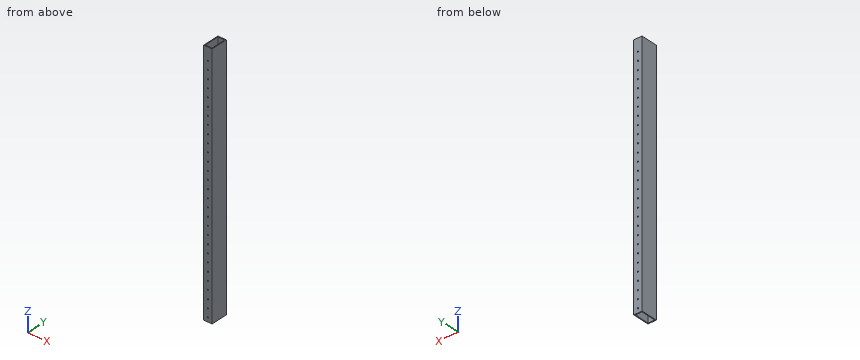
Autodesk Inventor part; units mm, degrees
ref_plane "YZ Plane" through (0, 0, 0) normal (1, 0, 0) x (0, 1, 0)
ref_plane "XZ Plane" through (0, 0, 0) normal (0, 1, 0) x (-1, 0, 0)
ref_plane "XY Plane" through (0, 0, 0) normal (0, 0, 1) x (1, 0, 0)
sketch "Sketch1" plane through (0, 0, 0) normal (0, 0, 1) x (1, 0, 0)
  line L0 (0, 0) -> (25.4, 0)
  line L1 (25.4, 0) -> (25.4, 50.8)
  line L2 (25.4, 50.8) -> (0, 50.8)
  line L3 (0, 50.8) -> (0, 0)
  line L4 (22.86, 48.26) -> (22.86, 2.54)
  line L5 (22.86, 2.54) -> (2.54, 2.54)
  line L6 (2.54, 2.54) -> (2.54, 48.26)
  line L7 (2.54, 48.26) -> (22.86, 48.26)
  dimension "d0" = 25.4
  dimension "d1" = 50.8
  dimension "d2" = 2.54
extrude "Extrusion1" add sketch "Sketch1" along normal blind 762
sketch "Sketch2" plane through (0, 50.8, 0) normal (0, 1, 0) x (1, 0, 0)
  circle A0 centre (12.7, -12.7) radius 1.9844
  line L0 (25.4, 0) -> (0, 0)
  line L1 (0, 0) -> (0, -762)
  circle A1 centre (12.7, -38.1) radius 1.9844
  circle A2 centre (12.7, -63.5) radius 1.9844
  circle A3 centre (12.7, -88.9) radius 1.9844
  circle A4 centre (12.7, -114.3) radius 1.9844
  circle A5 centre (12.7, -139.7) radius 1.9844
  circle A6 centre (12.7, -165.1) radius 1.9844
  circle A7 centre (12.7, -190.5) radius 1.9844
  circle A8 centre (12.7, -215.9) radius 1.9844
  circle A9 centre (12.7, -241.3) radius 1.9844
  circle A10 centre (12.7, -266.7) radius 1.9844
  circle A11 centre (12.7, -292.1) radius 1.9844
  circle A12 centre (12.7, -317.5) radius 1.9844
  circle A13 centre (12.7, -342.9) radius 1.9844
  circle A14 centre (12.7, -368.3) radius 1.9844
  circle A15 centre (12.7, -393.7) radius 1.9844
  circle A16 centre (12.7, -419.1) radius 1.9844
  circle A17 centre (12.7, -444.5) radius 1.9844
  circle A18 centre (12.7, -469.9) radius 1.9844
  circle A19 centre (12.7, -495.3) radius 1.9844
  circle A20 centre (12.7, -520.7) radius 1.9844
  circle A21 centre (12.7, -546.1) radius 1.9844
  circle A22 centre (12.7, -571.5) radius 1.9844
  circle A23 centre (12.7, -596.9) radius 1.9844
  circle A24 centre (12.7, -622.3) radius 1.9844
  circle A25 centre (12.7, -647.7) radius 1.9844
  circle A26 centre (12.7, -673.1) radius 1.9844
  circle A27 centre (12.7, -698.5) radius 1.9844
  circle A28 centre (12.7, -723.9) radius 1.9844
  circle A29 centre (12.7, -749.3) radius 1.9844
  circle A30 centre (12.7, -774.7) radius 1.9844
  circle A31 centre (12.7, -800.1) radius 1.9844
  circle A32 centre (12.7, -825.5) radius 1.9844
  dimension "d5" = 3.9688
  dimension "d6" = 12.7
  dimension "d7" = 12.7
  dimension "d10" = 25.4
extrude "Extrusion2" cut sketch "Sketch2" against normal blind 558.8 contours A0 | A1 | A2 | A3 | A4 | A5 | A6 | A7 | A8 | A9 | A10 | A11 | A12 | A13 | A14 | A15 | A16 | A17 | A18 | A19 | A20 | A21 | A22 | A23 | A24 | A25 | A26 | A27 | A28 | A30 | A31 | A32
properties part number "30in OChannel 1x2" material "Aluminum 6061-AHC"
Read the model definition and answer for the solid it produces. Units are mm, in the model's axes. Give positions to 0.01 mm unless a question says otherwise; leave off trailing zeros. Loops run counter-clockwise (first coordinate to the right, second up) from the corner with the lowest first, then second, coordinate; pieces in that order, holes last. Notation, with made-up numbers: M 77,34 L 121,34 A8 cw 121,40 Z; hole C 65.5,89.5 d10. An arc over 180 degrees is marked long. Write each question's results on one line, items separated by ' | '.
1. Given pin 1 (6.5 mm diameter, centred on x = 12.7, z = 38.1, fed in from -Y); pin 2 (3 mm diameter, centred on x = 12.7, z = 520.7, fed in from -Y), each flat-ended and moving along its own axis, determine where each tip first touches the part or whether it passes through.
Values:
pin 1: stops at y = 0 | pin 2: passes through
2. Section A-A on z = 632.5 is taken. Give the vertices of the cut face in (x, y), plus the area to 3 significant figures.
Values:
outline: M 0,0 L 25.4,0 L 25.4,50.8 L 0,50.8 Z; hole M 2.54,2.54 L 22.86,2.54 L 22.86,48.26 L 2.54,48.26 Z | area: 361 mm^2
3. Section B-B on y = 9.5 is taken. Give the vertices of the cut face in (x, z), plus the area to 3 significant figures.
Values:
outline: M 0,0 L 2.54,0 L 2.54,762 L 0,762 Z; M 22.86,0 L 25.4,0 L 25.4,762 L 22.86,762 Z | area: 3,870 mm^2
4. Straight lines are drawn through the part: line 1 (X direction, y = 3.5, z = 438.5); line 2 (Y direction, x = 16.5, z = 588); line 3 (X direction, y = 49.1, z = 495.3). For each, find the intervals that lie inside material, in ascending order. Write a range as [from, to].
Values:
line 1: x = [0, 2.54], [22.86, 25.4] | line 2: y = [0, 2.54], [48.26, 50.8] | line 3: x = [0, 10.72], [14.68, 25.4]
